Could you check a few things on this model? Use its own coordinates, in mm. A direction names the side the tool comes from. Coordinates: 2 decimals unless noted, no trailing zeros. Loops run counter-clockwise (first coordinate to the right, second up) from the corner with the lowest first, then second, coordinate; pieces in that order, holes last. Notation, with made-up numbers: (-19.75, 69) - (32.25, 69) arc R33 ccw to (32.25, 106) - close; hole circle Ø6 at (-7.5, 88). An arc over 180 degrees is marked (long way). One line per item, written item: value. Start each with the question number.
(1) If we section it at A-A on x = 0.85: Write out the boundary of the cut face in (y, z).
(2) If we mould it in two halves opening along Y, with no side actions, what happens to faces 1 (the face through (2.5, -1, 14)), 2 (the face through (0.035, 1.318, 22.126)), 3 (the face through (0.04, 0.71, 32.73))? For each: pulls with the +Y half, pulls with the -Y half, needs draft (parallel to the pull), parting line crosses it, or undercut.
(3) On a 3-axis mill with a long thin cutter (end or side, diameter ignored), from which of +Z, -Z, +X, -X, +Y, -Y can I reach the whole of each face in a straight line? I mean faces 4 (the face through (0.04, 4.3, 17.45)), 5 (the face through (0, 10, 0)), 6 (the face through (0, -10, 0)). Say none if no direction works.
(4) If we section it at D-D on z = 26: Write out the boundary of the cut face in (x, y), then the cut area to 4 significant figures.
(5) If we section it at C-C on z = 16: Write out the boundary of the cut face in (x, y), then the cut area to 3 significant figures.
(6) If we section it at B-B on y = 2.5: Write out the boundary of the cut face in (x, z).
(7) If I drill on line 1 along Y through (x, z) = (1.85, -0.5); line 2 along Y through (x, z) = (0.95, 19.5); line 3 along Y through (x, z) = (0.6, 15.5), over which ranges is the centre line in solid material (lowest first)? Write a range as from..to.
(8) I'm going to push flat-ended pins straight in: P1, Ø1.5, axis at x = 1.5, z = 20, coming from the -Y side; P2, Ø2, axis at x = -0.5, z = 5.5, coming from the +Y side; P3, Ø2.5, axis at x = -0.5, y = 9.5, coming from the -Z side. Where does each tip first touch, or does it pass through?
```python
from build123d import *

# Parameters (mm, degrees)
BOSS_EXTRUDE1_DEPTH = 2.5


with BuildPart() as part:
    # Sketch1 → Boss-Extrude1 (new, symmetric)
    with BuildSketch(Plane.YZ):
        with BuildLine():
            Line((-15.757717512, 0), (-5, 0))
            Line((-5, 0), (-5, -5))
            Line((-5, -5), (5, -5))
            Line((5, -5), (5, 0))
            Line((5, 0), (14.242282488, 0))
            Line((14.242282488, 0), (12.716235334, 20.927285791))
            ThreePointArc((12.716235334, 20.927285791), (0.446501859, 32.742179409), (-12.620138577, 21.815103933))
            Line((-12.620138577, 21.815103933), (-15.757717512, 0))
        make_face()
        Polygon((5.57894904, 19.645983596), (-3.064156301, 24.675569074), (-5.57894904, 20.354016404), (3.064156301, 15.324430926), align=None, mode=Mode.SUBTRACT)
    extrude(amount=BOSS_EXTRUDE1_DEPTH, both=True)


solid = part.part
```
Values:
1. outline: (-15.76, 0) - (-5, 0) - (-5, -5) - (5, -5) - (5, 0) - (14.24, 0) - (12.72, 20.93) arc R12.75 ccw to (-12.62, 21.82) - close; hole (-5.58, 20.35) - (3.06, 15.32) - (5.58, 19.65) - (-3.06, 24.68) - close
2. face 1: needs draft
2. face 2: undercut
2. face 3: parting line crosses it
3. face 4: +X, -X
3. face 5: -Z, +X, -X, +Y
3. face 6: -Z, +X, -X, -Y
4. outline: (-2.5, -11.25) - (2.5, -11.25) - (2.5, 11.25) - (-2.5, 11.25) - close
4. area: 112.5 mm2
5. outline: (-2.5, -13.46) - (2.5, -13.46) - (2.5, 1.9) - (-2.5, 1.9) - close; (-2.5, 3.46) - (2.5, 3.46) - (2.5, 13.08) - (-2.5, 13.08) - close
5. area: 125 mm2
6. outline: (-2.5, -5) - (2.5, -5) - (2.5, 15.65) - (-2.5, 15.65) - close; (-2.5, 21.44) - (2.5, 21.44) - (2.5, 32.5) - (-2.5, 32.5) - close
7. line 1: y = -5..5
7. line 2: y = -12.95..-4.11, 5.49..12.82
7. line 3: y = -13.53..2.76, 3.17..13.11
8. P1: stops at y = -12.99
8. P2: stops at y = 13.91
8. P3: stops at z = 0
